Geometry check sheet. Reference: the model listing, model coordinates, mm. A direction names the side the tool comes from. Coordinates: 2 decimals unless noted, no trailing zeros. Loops run counter-clockwise (first coordinate to the right, second up) from the corner with the lowest first, then second, coordinate; pieces in that order, holes last. Notation, with made-up numbers: (-30.5, 51) -> (14.5, 51) arc R23 ccw to (14.5, 89) -> close; hole circle Ø3 at (2.25, 48.5). An arc over 180 degrees is marked (long way). Answer as a JSON object with one key per item and string values.
from build123d import *

# Parameters (mm, degrees)
SKETCH_W     = 25.4
SKETCH_H     = 25.4
SKETCH_R     = 3.3782
PAD_DEPTH    = 2.032
SKETCH001_W  = 25.4
SKETCH001_H  = 25.4
SKETCH001_R  = 3.3782
PAD001_DEPTH = 2.032


with BuildPart() as part:
    # Sketch → Pad (new body)
    with BuildSketch(Plane.XY):
        Rectangle(SKETCH_W, SKETCH_H)
        Circle(SKETCH_R, mode=Mode.SUBTRACT)
    extrude(amount=PAD_DEPTH)

    # Sketch001 (on Face2 of Pad) → Pad001 (join)
    with BuildSketch(Plane.XZ.offset(12.7)):
        with Locations((0, -10.668)):
            Rectangle(SKETCH001_W, SKETCH001_H)
        with Locations((0, -10.668)):
            Circle(SKETCH001_R, mode=Mode.SUBTRACT)
    extrude(amount=-PAD001_DEPTH)


solid = part.part
1. Section check D-D, the plane x = 9.5. Record the boundary of the cut face in (y, z).
Evaluation:
{"outline": "(-12.7, -23.37) -> (-10.67, -23.37) -> (-10.67, 0) -> (12.7, 0) -> (12.7, 2.03) -> (-12.7, 2.03) -> close"}
2. Tool access check on faces 1 (the face through (3, -12.7, -8)), 2 (the face through (0, 4, 0)). Record the directions out of +Z, -Z, +X, -X, +Y, -Y that give a thin tool (end or side, any length) a straight path to the whole face; none if there is none.
Evaluation:
{"face 1": "+Z, -Z, +X, -X, -Y", "face 2": "-Z, +X, -X, +Y"}
3. Section check B-B, the plane y = 0. Record the boundary of the cut face in (x, z), then the cut area to 3 significant figures.
Evaluation:
{"outline": "(-12.7, 0) -> (-3.38, 0) -> (-3.38, 2.03) -> (-12.7, 2.03) -> close; (3.38, 0) -> (12.7, 0) -> (12.7, 2.03) -> (3.38, 2.03) -> close", "area": "37.9 mm^2"}
4. Depth check by flat-ended pin: P1, Ø4, axis at x = 1, z = -15, coming from the +Y side; P2, Ø2, axis at x = 6.5, y = 1, coming from the -Z side; P3, Ø10, axis at y = -2.5, z = -9.5, coming from the -X side. Enter the tip coordinate at first touch or a pass-through.
Evaluation:
{"P1": "stops at y = -10.67", "P2": "stops at z = 0", "P3": "passes through"}
5. Mould release check, pull along X, two halves, no side actions. Record for faces 3 (the face through (12.7, -11, -5)), 4 (the face through (-3, -10.668, -14)), 5 (the face through (-0.44, -11.7, -7.32)), 6 (the face through (-12.7, -11, -5)): released by +X, released by -X, zero draft, split by the parting line, or undercut.
Evaluation:
{"face 3": "released by +X", "face 4": "zero draft", "face 5": "undercut", "face 6": "released by -X"}
6. Thickness scan on probe 1 along Z at (x, y) = (0, -11.05); probe 2 along Y at (x, z) = (0, 1.2); probe 3 along Y at (x, z) = (-2.5, -5.5). Record the ranges inside material, lowest first. Write a range as from..to.
Evaluation:
{"probe 1": "z = -23.37..-14.05, -7.29..2.03", "probe 2": "y = -12.7..-3.38, 3.38..12.7", "probe 3": "y = -12.7..-10.67"}
7. Section check A-A, the plane x = 0. Record the boundary of the cut face in (y, z), then the cut area to 3 significant figures.
Evaluation:
{"outline": "(-12.7, -23.37) -> (-10.67, -23.37) -> (-10.67, -14.05) -> (-12.7, -14.05) -> close; (-12.7, -7.29) -> (-10.67, -7.29) -> (-10.67, 0) -> (-3.38, 0) -> (-3.38, 2.03) -> (-12.7, 2.03) -> close; (3.38, 0) -> (12.7, 0) -> (12.7, 2.03) -> (3.38, 2.03) -> close", "area": "71.6 mm^2"}
8. Section check C-C, the plane z = -12.75. Record the boundary of the cut face in (x, y).
Evaluation:
{"outline": "(-12.7, -12.7) -> (-2.66, -12.7) -> (-2.66, -10.67) -> (-12.7, -10.67) -> close; (2.66, -12.7) -> (12.7, -12.7) -> (12.7, -10.67) -> (2.66, -10.67) -> close"}
